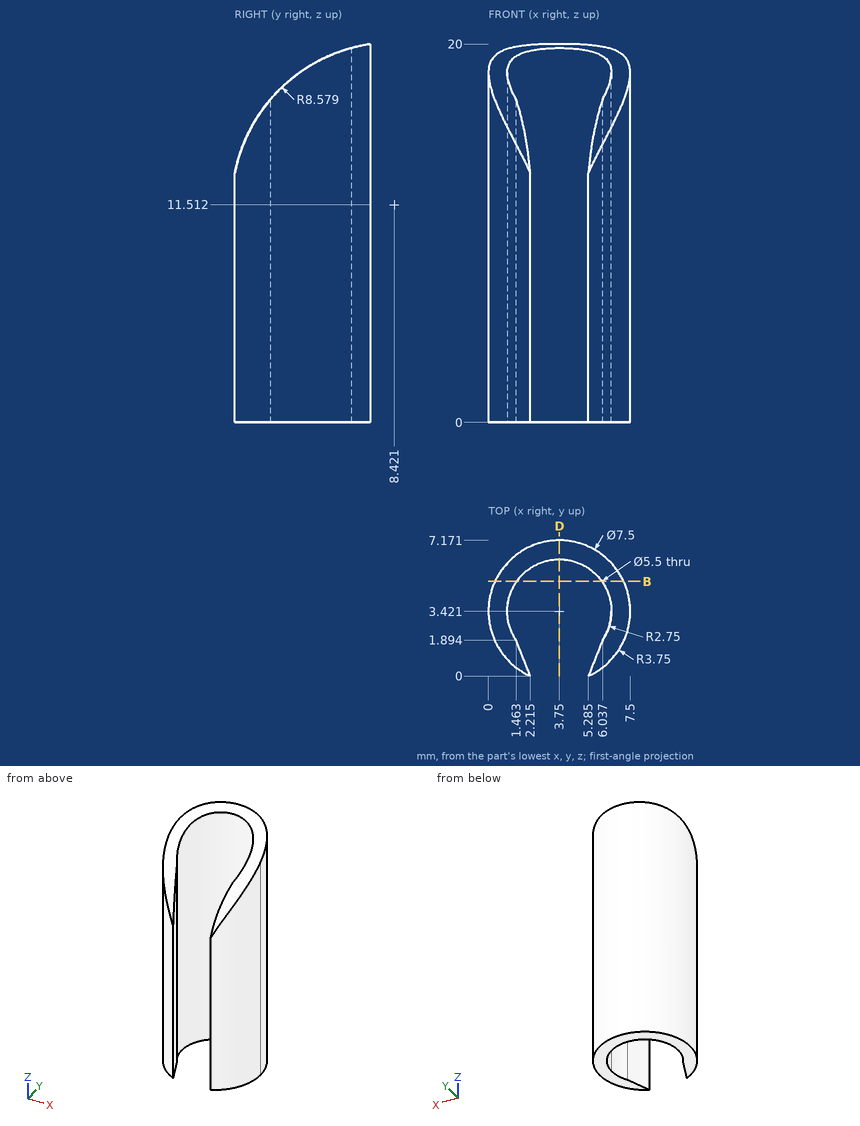
Geometry check sheet. Reference: drawing and pictorial views, mm from the part's lowest x, y, z. Round coordinates to 2 decimals unless told otherwise and drop trailing zeros. Order: outer loops, then holes, each group sorted by start corner. A loop starts at its lowest first (then second) coordinate and runs counter-clockwise, first axis right, second up. Notation, with made-up numbers: (1, 48) - (58, 48) arc R18 ccw to (58, 58) - close; hole circle Ø10 at (10.5, 71.25). An arc over 180 degrees is marked (long way). One line per question, with ' | ' between items. Start each with the question number.
(1) Sectioned sample at D-D on x = 3.75. Record the cut outline in (y, z), and give its area (3 significant figures).
(2) Sectioned sample at B-B on y = 5. Record the cut outline in (x, z).
(3) Thickness scan on L1, parallel to Y at x = 3.75, z = 5.5; L2, parallel to X at y = 1.5, z = 9.75; L3, parallel to X at y = 5.75, z = 16.5 (1 decimal). Record the ranges inside material, lowest first. Write a range as [from, to].
(4) Depth check by flat-ended pin: pin 1 Ø2 at (x, y) = (3.5, 5.5) entering from +Z; pin 2 Ø2 at (x, z) = (2.5, 12.5) entering from -Y; pin 3 Ø2 at (x, y) = (2, 2.5) entering from +Z; pin 4 Ø1.5 at (y, z) = (1.5, 16) entering from +X. Enter the tip coordinate at first touch or a pass-through.
Conclusion:
1) outline: (6.17, 0) - (7.17, 0) - (7.17, 20) arc R8.58 ccw to (6.17, 19.79) - close | area: 19.9 mm2
2) outline: (0.35, 0) - (1.5, 0) - (1.5, 19.38) - (0.35, 19.38) - close; (6, 0) - (7.15, 0) - (7.15, 19.38) - (6, 19.38) - close
3) L1: y = [6.17, 7.17] | L2: x = [0.53, 1.62], [5.88, 6.97] | L3: x = [0.8, 2.3], [5.2, 6.7]
4) pin 1: stops at z = 19.87 | pin 2: stops at y = 0 | pin 3: stops at z = 18.03 | pin 4: stops at x = 7.31
